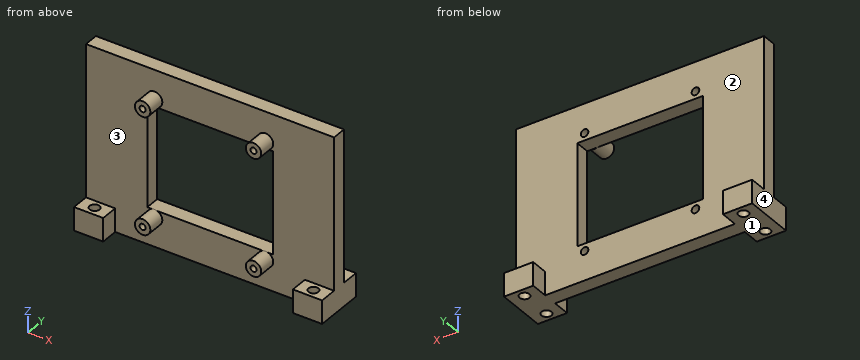
from build123d import *

# Parameters (mm, degrees)
SKETCH3_W           = 85
SKETCH3_H           = 60
BOSS_EXTRUDE3_DEPTH = 5
SKETCH5_W           = 43
SKETCH5_H           = 35
CUT_EXTRUDE2_DEPTH  = 10
CUT_EXTRUDE1_REACH  = 75.58
SKETCH4_R           = 1.3
SKETCH9_R           = 2.65
SKETCH9_R_2         = 1.05
BOSS_EXTRUDE5_DEPTH = 6
SKETCH10_W          = 10
SKETCH10_H          = 6
SKETCH10_R          = 1.7
BOSS_EXTRUDE6_DEPTH = 8


with BuildPart() as part:
    # Sketch3 → Boss-Extrude3 (new body)
    with BuildSketch(Plane(origin=(0, 0, 0), x_dir=(1, 0, 0), z_dir=(0, 1, 0))):
        with Locations((-24.5, 0)):
            Rectangle(SKETCH3_W, SKETCH3_H)
    extrude(amount=BOSS_EXTRUDE3_DEPTH)

    # Sketch5 → Cut-Extrude2 (cut)
    with BuildSketch(Plane.XZ):
        with Locations((-24.5, 0)):
            Rectangle(SKETCH5_W, SKETCH5_H)
    extrude(amount=-CUT_EXTRUDE2_DEPTH, mode=Mode.SUBTRACT)

    # Sketch4 → Cut-Extrude1 (cut, up to next)
    with BuildSketch(Plane(origin=(0, 5, 0), x_dir=(1, 0, 0), z_dir=(0, 1, 0)), mode=Mode.PRIVATE) as cut_extrude1_sk1:
        with Locations(Location((-43.5, 20, 0), (0, 0, 270))):
            Circle(SKETCH4_R)
    cut_extrude1_tool1 = extrude(cut_extrude1_sk1.sketch, amount=-CUT_EXTRUDE1_REACH, mode=Mode.PRIVATE) & part.part
    # Sketch4 → Cut-Extrude1 (cut, up to next)
    with BuildSketch(Plane(origin=(0, 5, 0), x_dir=(1, 0, 0), z_dir=(0, 1, 0)), mode=Mode.PRIVATE) as cut_extrude1_sk2:
        with Locations(Location((-5.5, 20, 0), (0, 0, 270))):
            Circle(SKETCH4_R)
    cut_extrude1_tool2 = extrude(cut_extrude1_sk2.sketch, amount=-CUT_EXTRUDE1_REACH, mode=Mode.PRIVATE) & part.part
    # Sketch4 → Cut-Extrude1 (cut, up to next)
    with BuildSketch(Plane(origin=(0, 5, 0), x_dir=(1, 0, 0), z_dir=(0, 1, 0)), mode=Mode.PRIVATE) as cut_extrude1_sk3:
        with Locations(Location((-5.5, -20, 0), (0, 0, 270))):
            Circle(SKETCH4_R)
    cut_extrude1_tool3 = extrude(cut_extrude1_sk3.sketch, amount=-CUT_EXTRUDE1_REACH, mode=Mode.PRIVATE) & part.part
    # Sketch4 → Cut-Extrude1 (cut, up to next)
    with BuildSketch(Plane(origin=(0, 5, 0), x_dir=(1, 0, 0), z_dir=(0, 1, 0)), mode=Mode.PRIVATE) as cut_extrude1_sk4:
        with Locations(Location((-43.5, -20, 0), (0, 0, 270))):
            Circle(SKETCH4_R)
    cut_extrude1_tool4 = extrude(cut_extrude1_sk4.sketch, amount=-CUT_EXTRUDE1_REACH, mode=Mode.PRIVATE) & part.part
    add(cut_extrude1_tool1.solids().sort_by_distance((-43.5, 5, -20))[0], mode=Mode.SUBTRACT)
    add(cut_extrude1_tool2.solids().sort_by_distance((-5.5, 5, -20))[0], mode=Mode.SUBTRACT)
    add(cut_extrude1_tool3.solids().sort_by_distance((-5.5, 5, 20))[0], mode=Mode.SUBTRACT)
    add(cut_extrude1_tool4.solids().sort_by_distance((-43.5, 5, 20))[0], mode=Mode.SUBTRACT)

    # Sketch9 → Boss-Extrude5 (add)
    # profile 1 of 4: a face of its own
    with BuildSketch(Plane.XZ):
        with Locations(Location((-43.5, 20, 0), (0, 0, 250.629961754))):
            Circle(SKETCH9_R)
        with Locations(Location((-43.5, 20, 0), (0, 0, 270))):
            Circle(SKETCH9_R_2, mode=Mode.SUBTRACT)
    # profile 2 of 4: a face of its own
    with BuildSketch(Plane.XZ):
        with Locations(Location((-43.5, -20, 0), (0, 0, 109.370038246))):
            Circle(SKETCH9_R)
        with Locations(Location((-43.5, -20, 0), (0, 0, 270))):
            Circle(SKETCH9_R_2, mode=Mode.SUBTRACT)
    # profile 3 of 4: a face of its own
    with BuildSketch(Plane.XZ):
        with Locations(Location((-5.5, 20, 0), (0, 0, 250.629961754))):
            Circle(SKETCH9_R)
        with Locations(Location((-5.5, 20, 0), (0, 0, 270))):
            Circle(SKETCH9_R_2, mode=Mode.SUBTRACT)
    # profile 4 of 4: a face of its own
    with BuildSketch(Plane.XZ):
        with Locations(Location((-5.5, -20, 0), (0, 0, 109.370038246))):
            Circle(SKETCH9_R)
        with Locations(Location((-5.5, -20, 0), (0, 0, 270))):
            Circle(SKETCH9_R_2, mode=Mode.SUBTRACT)
    extrude(amount=BOSS_EXTRUDE5_DEPTH)

    # Sketch10 → Boss-Extrude6 (add)
    # profile 1 of 4: a face of its own
    with BuildSketch(Plane(origin=(-17, 0, -30), x_dir=(-1, 0, 0), z_dir=(0, 0, -1))):
        with Locations((-30, -3)):
            Rectangle(SKETCH10_W, SKETCH10_H)
        with Locations((-30, -3)):
            Circle(SKETCH10_R, mode=Mode.SUBTRACT)
    # profile 2 of 4: a face of its own
    with BuildSketch(Plane(origin=(-17, 0, -30), x_dir=(-1, 0, 0), z_dir=(0, 0, -1))):
        with Locations((45, -3)):
            Rectangle(SKETCH10_W, SKETCH10_H)
        with Locations(Location((45, -3, 0), (0, 0, 180))):
            Circle(SKETCH10_R, mode=Mode.SUBTRACT)
    # profile 3 of 4: a face of its own
    with BuildSketch(Plane(origin=(-17, 0, -30), x_dir=(-1, 0, 0), z_dir=(0, 0, -1))):
        with Locations((45, 8)):
            Rectangle(SKETCH10_W, SKETCH10_H)
        with Locations((45, 8)):
            Circle(SKETCH10_R, mode=Mode.SUBTRACT)
    # profile 4 of 4: a face of its own
    with BuildSketch(Plane(origin=(-17, 0, -30), x_dir=(-1, 0, 0), z_dir=(0, 0, -1))):
        with Locations((-30, 8)):
            Rectangle(SKETCH10_W, SKETCH10_H)
        with Locations(Location((-30, 8, 0), (0, 0, 180))):
            Circle(SKETCH10_R, mode=Mode.SUBTRACT)
    extrude(amount=-BOSS_EXTRUDE6_DEPTH)


solid = part.part
Design review of the part built by this model. Coordinates are the model's own, in mm. Face numbers are marked on the shaded views. Round coordinates to 2 decimals unless told otherwise and drop trailing zeros. Write each loop counter-clockwise with the first axis right and the second up, starting at its lowest first coordinate (ties: lowest second). Pieces come first, ordered by that corner, then holes. Notation, with made-up numbers: (-34, 21.25) - (-26, 21.25) arc R15 cw to (-26, 25.25) - close; hole circle Ø10 at (57, 84). An arc over 180 degrees is marked (long way). Return JSON: item names as keys, results as strings. Group by question number.
Item 1: The part is to be moulded in two halves that separate along X. For the marked faces 1, 2, 3 and 4, say which applies: pulls with the +X half, pulls with the -X half, needs draft (parallel to the pull), parting line crosses it, or undercut.
Item 2: We need section B-B on y = 8. Write out the cut boundary in (x, z).
Item 3: We need section C-C on z = 20. Write out the cut boundary in (x, y), and give its area (3 significant figures).
Item 4: We need section A-A on x = -62. Write out the cut boundary in (y, z).
Item 5: We need section D-D on x = -32. Write out the cut boundary in (y, z), and give its area (3 significant figures).
Item 6: Insertion check: P1, Ø4.5, axis at x = -62, y = -3, coming from the +Z side; P2, Ø2.5, axis at x = -5.5, z = 20, coming from the -Y side; P3, Ø2.5, axis at x = -62, y = 8, coming from the +Z side; P4, Ø12, axis at x = 3, z = 1, coming from the +Y side. Each pin has a flat end and moves straight along its axis. Give the tip position at first contact, or say it passes through.
Item 7: For probe 1 along X at (y, z) = (3.9, -20); probe 2 along X at (y, z) = (-3.2, 20); probe 3 along Z at (x, y) = (-33, 2.5), list the stretches that pass through material, from the lowest coordinate up. Write a range as [from, to].
Model answer:
{
 "1": {"face 1": "needs draft", "face 2": "undercut", "face 3": "undercut", "face 4": "pulls with the -X half"},
 "2": {"outline": "(-67, -30) - (-63.7, -30) - (-63.7, -22) - (-67, -22) - close; (-60.3, -30) - (-57, -30) - (-57, -22) - (-60.3, -22) - close; (8, -30) - (11.3, -30) - (11.3, -22) - (8, -22) - close; (14.7, -30) - (18, -30) - (18, -22) - (14.7, -22) - close"},
 "3": {"outline": "(-67, 0) - (-46.15, 0) - (-46.15, -6) - (-44.55, -6) - (-44.55, 0) - (-44.8, 0) - (-44.8, 5) - (-67, 5) - close; (-42.45, -6) - (-40.85, -6) - (-40.85, 0) - (-8.15, 0) - (-8.15, -6) - (-6.55, -6) - (-6.55, 0) - (-6.8, 0) - (-6.8, 5) - (-42.2, 5) - (-42.2, 0) - (-42.45, 0) - close; (-4.45, -6) - (-2.85, -6) - (-2.85, 0) - (18, 0) - (18, 5) - (-4.2, 5) - (-4.2, 0) - (-4.45, 0) - close", "area": "437 mm²"},
 "4": {"outline": "(-6, -30) - (-4.7, -30) - (-4.7, -22) - (-6, -22) - close; (-1.3, -30) - (6.3, -30) - (6.3, -22) - (5, -22) - (5, 30) - (0, 30) - (0, -22) - (-1.3, -22) - close; (9.7, -30) - (11, -30) - (11, -22) - (9.7, -22) - close"},
 "5": {"outline": "(0, -30) - (5, -30) - (5, -17.5) - (0, -17.5) - close; (0, 17.5) - (5, 17.5) - (5, 30) - (0, 30) - close", "area": "125 mm²"},
 "6": {"P1": "stops at z = -22", "P2": "stops at y = -6", "P3": "passes through", "P4": "stops at y = 5"},
 "7": {"probe 1": "x = [-67, -44.8], [-42.2, -6.8], [-4.2, 18]", "probe 2": "x = [-46.15, -44.55], [-42.45, -40.85], [-8.15, -6.55], [-4.45, -2.85]", "probe 3": "z = [-30, -17.5], [17.5, 30]"}
}
